Study the drawing (mm; zero at the part's minimum x, y, z) and answer. A direction names the side the tool comes from. Give positions to 0.01 mm unless a question says otherwise; leave off trailing zeros. Order: outer loops, then holes, each group sorted by start corner. A loop starts at its lowest first (then second) coordinate and runs counter-clockwise, first axis right, second up. Notation, with made-up numbers: (-4.75, 66) - (27.25, 66) arc R16 cw to (27.25, 77) - close; hole circle Ø2 at (-17.75, 33). An arc over 180 degrees is marked (long way). Write each question's results on one line, items separated by ' | '. Start each with the question number.
Q1. Find section C-C on x = 26.5. Give the vertices of the cut face in (y, z) (3 decimals), and give its area (3 significant figures).
Q2. Find section D-D on x = 3.5. Give the vertices of the cut face in (y, z).
Q3. Find the intervals of material crossed by line 1 along Y through (x, z) = (39, 2); line 2 along Z through (x, y) = (35.5, 49.5); line 3 along X through (y, z) = (21.5, 0.5), in increasing order. Write a range as from..to.
Q4. Find section B-B on y = 22.5. Give the vertices of the cut face in (x, z), and give its area (3 significant figures).
Q5. Flat-ended cylindrical pins translate along their axes: P1, Ø0.5, axis at y = 46, z = 1, coming from the +X side; P2, Ø1.8, axis at y = 44.5, z = 1, coming from the -X side; P3, Ø23, axis at x = 14.5, y = 20.5, coming from the +Z side. Find the tip coordinate at first contact, or state that the pin passes through.
Q6. Find section A-A on z = 1. Give the vertices of the cut face in (x, y).
Q7. A tool of negligible diameter and unlimited length cuts with its end or side. For the marked faces 1 and 2, from which of +Z, -Z, +X, -X, +Y, -Y can it reach the whole face along a straight path? Write none if from no direction.
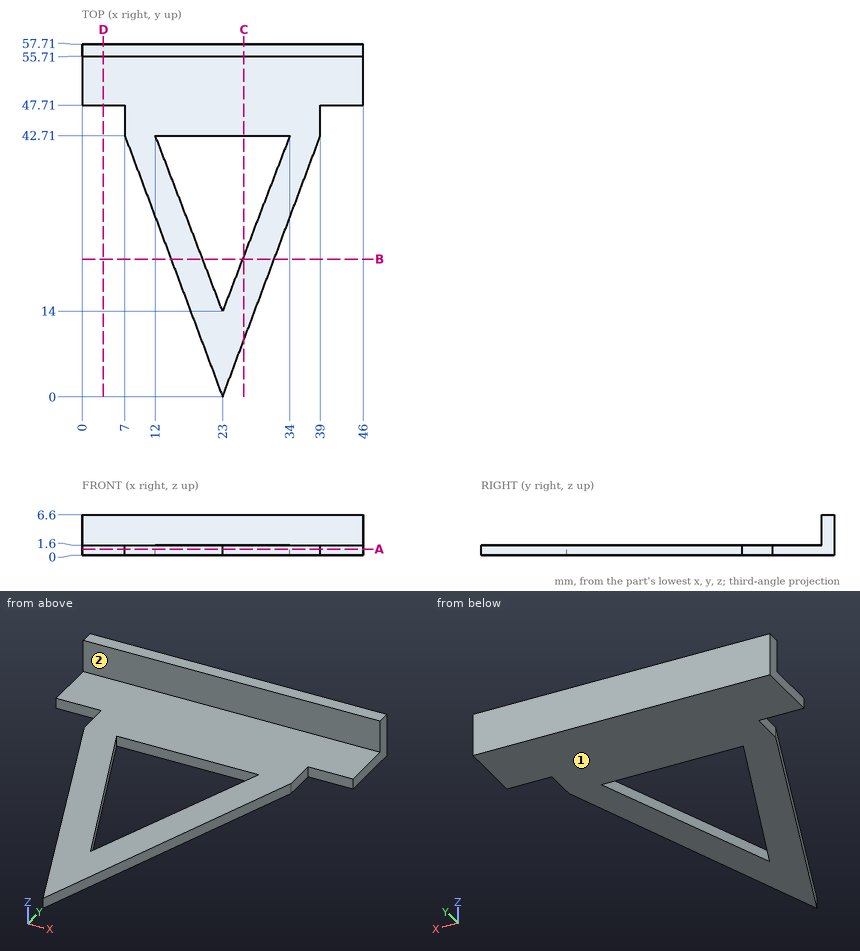
Working result:
1) outline: (9.343, 0) - (23.135, 0) - (23.135, 1.6) - (9.343, 1.6) - close; (42.71, 0) - (57.71, 0) - (57.71, 6.6) - (55.71, 6.6) - (55.71, 1.6) - (42.71, 1.6) - close | area: 56.1 mm²
2) outline: (47.71, 0) - (57.71, 0) - (57.71, 6.6) - (55.71, 6.6) - (55.71, 1.6) - (47.71, 1.6) - close
3) line 1: 55.71..57.71 | line 2: 0..1.6 | line 3: 14.95..20.13, 25.87..31.05
4) outline: (14.57, 0) - (19.74, 0) - (19.74, 1.6) - (14.57, 1.6) - close; (26.26, 0) - (31.43, 0) - (31.43, 1.6) - (26.26, 1.6) - close | area: 16.6 mm²
5) P1: x = 39 | P2: x = 7 | P3: z = 1.6
6) outline: (0, 47.71) - (7, 47.71) - (7, 42.71) - (23, 0) - (39, 42.71) - (39, 47.71) - (46, 47.71) - (46, 57.71) - (0, 57.71) - close; hole (12, 42.71) - (23, 14) - (34, 42.71) - close
7) face 1: -Z, +X, -X, +Y, -Y | face 2: +Z, +X, -X, -Y
